from build123d import *

# Parameters (mm, degrees)
F0_W     = 200
F0_H     = 100
F1_DEPTH = 10
F2_W     = 198
F2_H     = 98
F3_DEPTH = 2
F4_W     = 50
F4_H     = 40
F5_DEPTH = 10
F6_R     = 5
F7_DEPTH = 5


with BuildPart() as f1:
    # F0 (on Front) → F1 (new body)
    with BuildSketch(Plane.XZ):
        with Locations((0, -12.41183)):
            Rectangle(F0_W, F0_H)
    extrude(amount=F1_DEPTH)

    # F2 (on face) → F3 (cut)
    with BuildSketch(Plane.XZ.offset(10)):
        with Locations((0, -12.41183)):
            Rectangle(F2_W, F2_H)
    extrude(amount=-F3_DEPTH, mode=Mode.SUBTRACT)

    # F4 (on face) → F5 (join)
    with BuildSketch(Plane(origin=(0, 0, 0), x_dir=(-1, 0, 0), z_dir=(0, 1, 0))):
        with Locations((-0.960992, -7.41183)):
            Rectangle(F4_W, F4_H)
    extrude(amount=F5_DEPTH)

    # F6 (on face) → F7 (join)
    with BuildSketch(Plane(origin=(0, 10, 0), x_dir=(-1, 0, 0), z_dir=(0, 1, 0))):
        Circle(F6_R)
    extrude(amount=F7_DEPTH)


solid = f1.part
The model under review builds one solid part; all positions refer to its coordinate system, in mm. A direction names the side the tool comes from. Give positions to 0.01 mm unless a question says otherwise; leave off trailing zeros. Write each loop counter-clockwise with the first axis right and the second up, starting at its lowest first coordinate (ties: lowest second). Pieces come first, ordered by that corner, then holes.
1. For P1, Ø20, axis at x = -7.5, z = -14, coming from the +Y side; P2, Ø11, axis at y = 5, z = 1.5, coming from the -X side; P3, Ø3, axis at x = 3, y = 3.5, coming from the +Z side; P4, Ø5, axis at x = 4.5, y = 6, coming from the -Z side, all flat-tipped, find the tip position at first contact; note any pin that passes through.
2. Add section B-B, the plane z = 28.5. Write out the cut boundary in (x, y).
3. Add section D-D, the plane y = 5. Write out the cut boundary in (x, z), plus the area to 3 significant figures.
4. Wall thickness on L1, parallel to Y at x = 62, z = -29; L2, parallel to Y at x = -17, z = 6; L3, parallel to X at y = -8.25, z = 22: over which ranges is each line inside the solid? List them lowest first.
5. Add section A-A, the plane x = 0. Write out the cut boundary in (y, z).
6. Add section C-C, the plane x = 61. Write out the cut boundary in (y, z), plus the area to 3 significant figures.
7. Tool access review of faces 1 (the flat face through (1, 5, 12.588)), 2 (the flat face through (-100, -5, -13)), 3 (the flat face through (1, 5, -27.412)), 4 (the flat face through (25.961, 5, -8)), 5 (the cylindrical face through (1.08, 12.46, -4.88)): name each direction out of +Z, -Z, +X, -X, +Y, -Y from which nothing blocks a thin tool from reaching the whole face with its end or side.
8. Draft analysis for pull direction X (two halves, no side actions). For faces 6 (the flat face through (-24.039, 5, -8)), 7 (the flat face through (-1, -8, -12)), 8 (the flat face through (-1, 0, -34)), state which applies: +X half, -X half, draft (parallel to the pull), parting line (faces both ways), or undercut.
Worked answers:
1. P1: stops at y = 10
1. P2: stops at x = -100
1. P3: stops at z = 12.59
1. P4: stops at z = -27.41
2. outline: (-100, -10) - (-99, -10) - (-99, -8) - (99, -8) - (99, -10) - (100, -10) - (100, 0) - (-100, 0) - close
3. outline: (-24.04, -27.41) - (25.96, -27.41) - (25.96, 12.59) - (-24.04, 12.59) - close
3. area: 2,000 mm2
4. L1: y = -8 to 0
4. L2: y = -8 to 10
4. L3: x = -100 to -99, 99 to 100
5. outline: (-10, -62.41) - (0, -62.41) - (0, -27.41) - (10, -27.41) - (10, -5) - (15, -5) - (15, 5) - (10, 5) - (10, 12.59) - (0, 12.59) - (0, 37.59) - (-10, 37.59) - (-10, 36.59) - (-8, 36.59) - (-8, -61.41) - (-10, -61.41) - close
6. outline: (-10, -62.41) - (0, -62.41) - (0, 37.59) - (-10, 37.59) - (-10, 36.59) - (-8, 36.59) - (-8, -61.41) - (-10, -61.41) - close
6. area: 804 mm2
7. face 1: +Z, +X, -X, +Y
7. face 2: +Z, -Z, -X, +Y, -Y
7. face 3: -Z, +X, -X, +Y
7. face 4: +Z, -Z, +X, +Y
7. face 5: +Y
8. face 6: -X half
8. face 7: undercut
8. face 8: draft
